Could you check a few things on this model? Use its own coordinates, in mm. Round coordinates to 2 decimals unless told otherwise and drop trailing zeros. Loops run counter-clockwise (first coordinate to the right, second up) from the corner with the lowest first, then second, coordinate; pieces in that order, holes last. Notation, with made-up numbers: M 5.25,12 L 21.25,12 A21 ccw 21.25,43 Z; hole C 48.5,37 d9. An arc over 180 degrees is marked long. Answer in a Markdown table with one row per item.
Autodesk Inventor part; units mm, degrees
ref_plane "YZ Plane" through (0, 0, 0) normal (1, 0, 0) x (0, 1, 0)
ref_plane "XZ Plane" through (0, 0, 0) normal (0, 1, 0) x (-1, 0, 0)
ref_plane "XY Plane" through (0, 0, 0) normal (0, 0, 1) x (1, 0, 0)
sketch "Sketch1" plane through (0, 0, 0) normal (0, 0, 1) x (1, 0, 0)
  line L0 (0, 0) -> (0, -161.1088)
  line L1 (0, 0) -> (244.475, 0)
  line L2 (244.475, 0) -> (244.475, -161.1088)
  line L3 (349.4217, -286.1793) -> (527.05, -317.5)
  line L4 (527.05, -317.5) -> (527.05, -565.7464)
  line L5 (527.05, -565.7464) -> (306.969, -526.9402)
  arc A0 (244.475, -161.1088) -> (349.4217, -286.1793) centre (371.475, -161.1088) ccw
  arc A1 (0, -161.1088) -> (306.969, -526.9402) centre (371.475, -161.1088) ccw
  dimension "d0" = 244.475
  dimension "d1" = 244.475
  dimension "d2" = 100
  dimension "d3" = 127
  dimension "d4" = 371.475
  dimension "d5" = 317.5
  dimension "d6" = 527.05
extrude "Extrusion1" add sketch "Sketch1" along normal blind 6.35
sketch "Sketch2" plane through (0, 0, 6.35) normal (0, 0, 1) x (1, 0, 0)
  line L0 (0, 0) -> (244.475, 0)
  line L1 (0, -161.1088) -> (0, 0)
  arc A0 (0, -161.1088) -> (306.969, -526.9402) centre (371.475, -161.1088) ccw
  line L2 (527.05, -565.7464) -> (306.969, -526.9402)
  line L3 (527.05, -317.5) -> (527.05, -565.7464)
  line L4 (349.4217, -286.1793) -> (527.05, -317.5)
  arc A1 (244.475, -161.1088) -> (349.4217, -286.1793) centre (371.475, -161.1088) ccw
  line L5 (244.475, 0) -> (244.475, -161.1088)
  arc A2 (239.7125, -161.1088) -> (348.5947, -290.8695) centre (371.475, -161.1088) ccw
  line L6 (348.5947, -290.8695) -> (527.05, -322.336)
  line L7 (527.05, -560.9105) -> (307.796, -522.2501)
  arc A3 (4.7625, -161.1088) -> (307.796, -522.2501) centre (371.475, -161.1088) ccw
  line L8 (4.7625, -161.1088) -> (4.7625, 0)
  line L9 (239.7125, 0) -> (239.7125, -161.1088)
  line L10 (7.9375, 0) -> (7.9375, -161.1088)
  arc A4 (7.9375, -161.1088) -> (308.3474, -519.1233) centre (371.475, -161.1088) ccw
  line L11 (308.3474, -519.1233) -> (527.05, -557.6865)
  line L12 (236.5375, 0) -> (236.5375, -161.1088)
  arc A5 (236.5375, -161.1088) -> (348.0433, -293.9962) centre (371.475, -161.1088) ccw
  line L13 (348.0433, -293.9962) -> (527.05, -325.5599)
  line L14 (4.7625, 0) -> (7.9375, 0)
  line L15 (239.7125, 0) -> (236.5375, 0)
  line L16 (527.05, -322.336) -> (527.05, -325.5599)
  line L17 (527.05, -560.9105) -> (527.05, -557.6865)
  dimension "d9" = 4.7625
  dimension "d10" = 4.7625
  dimension "d11" = 4.7625
  dimension "d12" = 4.7625
  dimension "d13" = 4.7625
  dimension "d14" = 4.7625
  dimension "d15" = 3.175
  dimension "d16" = 3.175
  dimension "d17" = 3.175
  dimension "d18" = 3.175
extrude "Extrusion2" cut sketch "Sketch2" against normal blind 3.175 contours L0 L10 A4 L11 L3 L7 A3 L8 | L0 L9 A2 L6 L3 L13 A5 L12
hole "Hole1" at (496.8748, -377.825, 6.35) direction (0, 0, -1) diameter 6.731 depth 25.4 tip angle 118
pattern_linear "Rectangular Pattern1" count 2 spacing 127 along (0, -1, 0) of "Hole1"
hole "Hole2" at (200.025, -12.7, 6.35) direction (0, 0, -1) diameter 6.731 depth 25.4 tip angle 118
pattern_linear "Rectangular Pattern2" count 3 spacing 76.2 along (-1, 0, 0) of "Hole2"
equation "\"d1\" = d0"
equation "\"d4\" = d3 + d0"
equation "\"d9\" = d10"
equation "\"d11\" = d10"
equation "\"d12\" = d10"
equation "\"d13\" = d10"
equation "\"d14\" = d10"
properties part number "GE-12070-01"
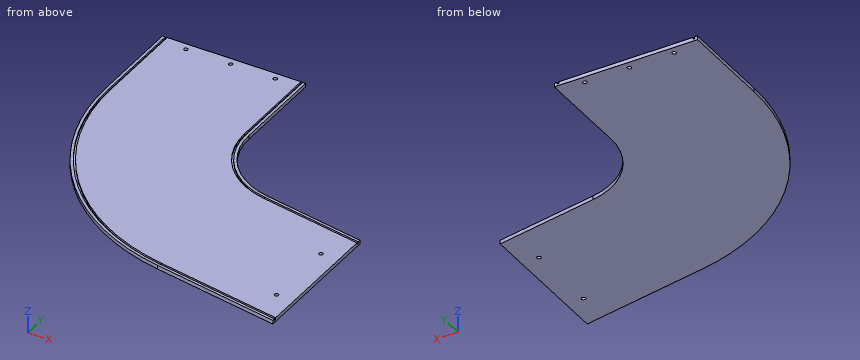
1) I want a section at C-C, the plane x = 67.5. Please give me the cut outline in (y, z) (3 decimals), plus the area to 3 significant figures.
Computed:
| item | result |
|---|---|
| outline | M -374.634,0 L 0,0 L 0,6.35 L -360.505,6.35 L -360.505,3.175 L -366.236,3.175 L -366.236,6.35 L -374.634,6.35 Z |
| area | 2,360 mm² |
2) I want a section at D-D, the plane x = 403. Please give me the cut outline in (y, z) (3 decimals), plus the area to 3 significant figures.
Computed:
| item | result |
|---|---|
| outline | M -543.873,0 L -295.627,0 L -295.627,6.35 L -300.463,6.35 L -300.463,3.175 L -303.687,3.175 L -303.687,6.35 L -535.813,6.35 L -535.813,3.175 L -539.037,3.175 L -539.037,6.35 L -543.873,6.35 Z |
| area | 1,560 mm² |
3) Will these pins go through, and if not, where does the flat tip stop? P1, Ø2.5, axis at y = -109, z = 5, coming from the +X side (3 decimals); P2, Ø2, axis at x = 458, z = 1.5, coming from the +Y side.
Computed:
| item | result |
|---|---|
| P1 | stops at x = 244.475 |
| P2 | stops at y = -305.15 |
4) I want a section at A-A, the plane z = 4.5. State how many separate pieces and enclosed holes the cut face has, plus the area to 3 significant figures.
Computed:
| item | result |
|---|---|
| separate pieces | 3 |
| enclosed holes | 5 |
| area | 169,000 mm² |
5) I need wall thicknesses on line 1 (X direction, y = -77.5, z = 5) (1 decimal); line 2 (X direction, y = -12.7, z = 4.5) (1 decimal); line 3 (Y direction, x = 309.5, z = 4.5). Which ranges of each line are inside material? Lowest first, please.
Computed:
| item | result |
|---|---|
| line 1 | x = 0 to 4.8, 7.9 to 236.5, 239.7 to 244.5 |
| line 2 | x = 0 to 4.8, 7.9 to 44.3, 51 to 120.5, 127.2 to 196.7, 203.4 to 236.5, 239.7 to 244.5 |
| line 3 | y = -527.39 to -522.55, -519.33 to -280.97, -277.39 to -271.96 |
